The listing builds one solid part. Answer for the finished solid, in the listing's coordinates (mm). A direction names the side the tool comes from. Give positions to 0.01 mm unless a question says otherwise; leave off trailing zeros. Loops run counter-clockwise (first coordinate to the right, second up) from the corner with the lowest first, then second, coordinate; pieces in that order, holes last. Notation, with made-up numbers: (23.5, 51.5) -> (54.5, 51.5) arc R18 cw to (54.5, 63.5) -> close; hole circle Ø4 at (68, 2). An arc over 180 degrees is marked (long way). One line per question, with ' | ' between items. Start each with the question number.
from build123d import *

# Parameters (mm, degrees)
F0_R     = 15
F0_R_2   = 14
F1_DEPTH = 124
F3_W     = 6.176928
F3_H     = 5.5
F4_DEPTH = 6


with BuildPart() as f1:
    # F0 (on Front) → F1 (new body)
    with BuildSketch(Plane.XZ):
        Circle(F0_R)
        Circle(F0_R_2, mode=Mode.SUBTRACT)
    extrude(amount=-F1_DEPTH)

    # F3 (on offset) → F4 (join)
    with BuildSketch(Plane.XZ.offset(-20)):
        with Locations((11.088464, 0)):
            Rectangle(F3_W, F3_H)
    extrude(amount=-F4_DEPTH)


solid = f1.part
1. The part is cut by section D-D (z = 4.75). Write down the section's boundary in (x, y).
2. Each of these flat-tipped pins is pushed along its axis until it touches: pin 1 Ø3 at (x, z) = (10.5, 1.5) entering from -Y; pin 2 Ø10 at (x, z) = (6.5, 4.5) entering from +Y; pin 3 Ø6 at (y, z) = (43, 10.5) entering from -X; pin 4 Ø3 at (x, y) = (0.5, 29.5) entering from -Z. Where does it stop, or does it pass through?
3. Determine the mould class of faces 1 (the cylindrical face through (-14.985, 61.132, 0.66)), 2 (the flat face through (11, 26, 0)) for opening direction Z: released by +Z, released by -Z, zero draft, split by the parting line, or undercut.
4. The part is cut by section B-B (z = 0). Write down the section's boundary in (x, y), plus the area to 3 significant figures.
5. The part is cut by section A-A (x = 0). Write down the section's boundary in (y, z).
6. For faces 3 (the flat face through (8, 23, 0)), 4 (the flat face through (11, 20, 0)), determine the directions among +Z, -Z, +X, -X, +Y, -Y from which every point of the face is accessible in a straight line to the end or side of a thin tool.
7. Straight lines are drawn through the part: L1, parallel to Z at x = 0, y = 72; L2, parallel to Y at x = 10.75, z = 2; L3, parallel to Z at x = -10.5, y = 96. For each, find the intervals that lie inside material, in ascending order.
8. The part is cut by section C-C (y = 95.5). Write down the section's boundary in (x, z).
Check sheet entries:
1) outline: (-14.23, 0) -> (-13.17, 0) -> (-13.17, 124) -> (-14.23, 124) -> close; (13.17, 0) -> (14.23, 0) -> (14.23, 124) -> (13.17, 124) -> close
2) pin 1: stops at y = 20 | pin 2: stops at y = 26 | pin 3: stops at x = -12.99 | pin 4: stops at z = -15
3) face 1: split by the parting line | face 2: undercut
4) outline: (-15, 0) -> (-14, 0) -> (-14, 124) -> (-15, 124) -> close; (8, 20) -> (14, 20) -> (14, 0) -> (15, 0) -> (15, 124) -> (14, 124) -> (14, 26) -> (8, 26) -> close | area: 284 mm^2
5) outline: (0, -15) -> (124, -15) -> (124, -14) -> (0, -14) -> close; (0, 14) -> (124, 14) -> (124, 15) -> (0, 15) -> close
6) face 3: +Y, -Y | face 4: -Y
7) L1: z = -15 to -14, 14 to 15 | L2: y = 20 to 26 | L3: z = -10.71 to -9.26, 9.26 to 10.71
8) outline: circle Ø30 at (0, 0); hole circle Ø28 at (0, 0)
